The model under review builds one solid part; all positions refer to its coordinate system, in mm. Face numbers are marked on the shaded views. A direction names the side the tool comes from. Round coordinates to 2 decimals unless told otherwise and drop trailing zeros. Order: outer loops, then holes, each group sorted by start corner. A loop starts at its lowest first (then second) coordinate and runs counter-clockwise, first axis right, second up.
1) Machinability: for the marked faces 1 and 2, which of the approach directions +Z, -Z, +X, -X, +Y, -Y give a long, thin tool a straight path to every point of the face, cutting with its end or side? Answer none if there is none.
2) Consider section D-D (x = 2). Give the boundary of the cut face in (y, z) (3 decimals), then the cut area to 3 significant figures.
3) Clearance check with flat-ended pins moving along their axes: P1, Ø6, axis at x = 17.5, y = 8.5, coming from the +Z side (3 decimals); P2, Ø1, axis at y = 2.5, z = -6, coming from the +X side; P3, Ø2, axis at x = 14.5, z = -18, coming from the +Y side. State where each tip first meets the part, or that it passes through.
4) Consider section C-C (z = -20.5). Give the boundary of the cut face in (x, y) (3 decimals), then the cut area to 3 significant figures.
5) Mouldability with a two-part tool opening along Y and no side actions: class the marked faces 3, 4 and 5 as pulls with the +Y half, pulls with the -Y half, needs draft (parallel to the pull), parting line crosses it, or undercut.
6) Consider section B-B (y = 13.25). Give the boundary of the cut face in (x, z) (3 decimals).
7) Consider section A-A (z = -3.81). Give the boundary of the cut face in (x, y).
8) To check wall thickness, follow L1, parallel to Z at x = 6.5, y = 9 (3 decimals); L2, parallel to Z at x = 2.25, y = 10.25 (3 decimals); L3, parallel to X at y = 15.75, z = -5. State the ranges of each line that lie inside material, in increasing order.
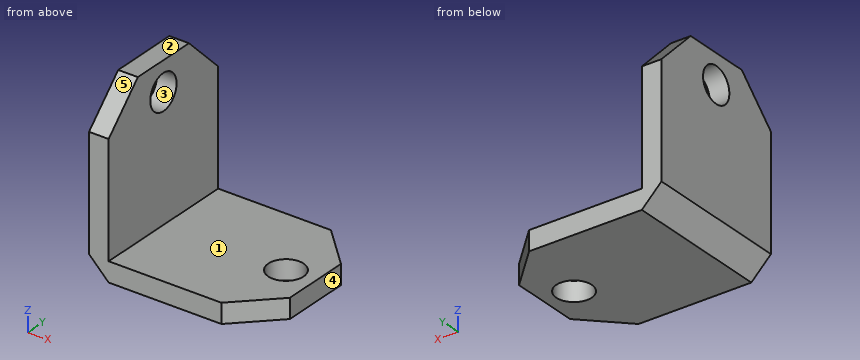
from build123d import *

# Parameters (mm, degrees)
BOSS_EXTRUDE1_DEPTH = 19.05
SKETCH2_R           = 2.286
CUT_EXTRUDE1_DEPTH  = 2.54
SKETCH3_R           = 2.286
CUT_EXTRUDE2_DEPTH  = 2.54
CHAMFER1_SIZE       = 5.08
CHAMFER2_SIZE       = 2.54


with BuildPart() as part:
    # Sketch1 → Boss-Extrude1 (new body)
    with BuildSketch(Plane(origin=(0, 0, 0), x_dir=(1, 0, 0), z_dir=(0, 1, 0))):
        Polygon((22.225, 22.225), (22.225, 19.685), (2.54, 19.685), (2.54, 0), (0, 0), (0, 22.225), align=None)
    extrude(amount=BOSS_EXTRUDE1_DEPTH)

    # Sketch2 → Cut-Extrude1 (cut)
    with BuildSketch(Plane.XY.offset(-19.685)):
        with Locations((18.415, 9.525)):
            Circle(SKETCH2_R)
    extrude(amount=-CUT_EXTRUDE1_DEPTH, mode=Mode.SUBTRACT)

    # Sketch3 → Cut-Extrude2 (cut)
    with BuildSketch(Plane(origin=(2.54, 0, 0), x_dir=(0, 0, -1), z_dir=(1, 0, 0))):
        with Locations((3.81, 9.525)):
            Circle(SKETCH3_R)
    extrude(amount=-CUT_EXTRUDE2_DEPTH, mode=Mode.SUBTRACT)

    # Chamfer1
    chamfer1_edges = [part.edges().sort_by_distance(p)[0] for p in [
        (22.225, 0, -20.955),
        (1.27, 19.05, 0),
        (22.225, 19.05, -20.955),
        (1.27, 0, 0),
    ]]
    chamfer(chamfer1_edges, length=CHAMFER1_SIZE)

    # Chamfer2
    chamfer2_edges = [part.edges().sort_by_distance(p)[0] for p in [
        (0, 9.525, -22.225),
    ]]
    chamfer(chamfer2_edges, length=CHAMFER2_SIZE)


solid = part.part
Answer below:
1. face 1: +Z, +X, +Y, -Y
1. face 2: +Z, +X, -X, +Y, -Y
2. outline: (0, -21.685) - (19.05, -21.685) - (19.05, -5.08) - (13.97, 0) - (5.08, 0) - (0, -5.08) - close; hole circle Ø4.572 at (9.525, -3.81)
2. area: 371 mm2
3. P1: stops at z = -19.685
3. P2: stops at x = 2.54
3. P3: passes through
4. outline: (0.815, 0) - (17.145, 0) - (22.225, 5.08) - (22.225, 13.97) - (17.145, 19.05) - (0.815, 19.05) - close; hole circle Ø4.572 at (18.415, 9.525)
4. area: 366 mm2
5. face 3: undercut
5. face 4: needs draft
5. face 5: pulls with the -Y half
6. outline: (0, -19.685) - (2.54, -22.225) - (22.225, -22.225) - (22.225, -19.685) - (2.54, -19.685) - (2.54, 0) - (0, 0) - close
7. outline: (0, 1.27) - (2.54, 1.27) - (2.54, 7.24) - (0, 7.24) - close; (0, 11.81) - (2.54, 11.81) - (2.54, 17.78) - (0, 17.78) - close
8. L1: z = -22.225 to -19.685
8. L2: z = -21.935 to -5.978, -1.642 to 0
8. L3: x = 0 to 2.54
